For this review, use the dimensioned drawing (mm, ordinates from the lowest corner) and the shaded views. A direction names the side the tool comes from. Round coordinates to 2 decimals unless told otherwise and drop trailing zeros. Order: outer loops, then holes, each group sorted by start corner. A loop starts at its lowest first (then second) coordinate and runs counter-clockwise, first axis right, second up. Notation, with made-up numbers: (-31, -31.5) -> (5, -31.5) arc R31 cw to (5, -4.5) -> close; hole circle Ø11 at (-2.5, 31.5). An arc over 180 degrees is marked (long way). Use a Markdown table: item, result. Add a question column.
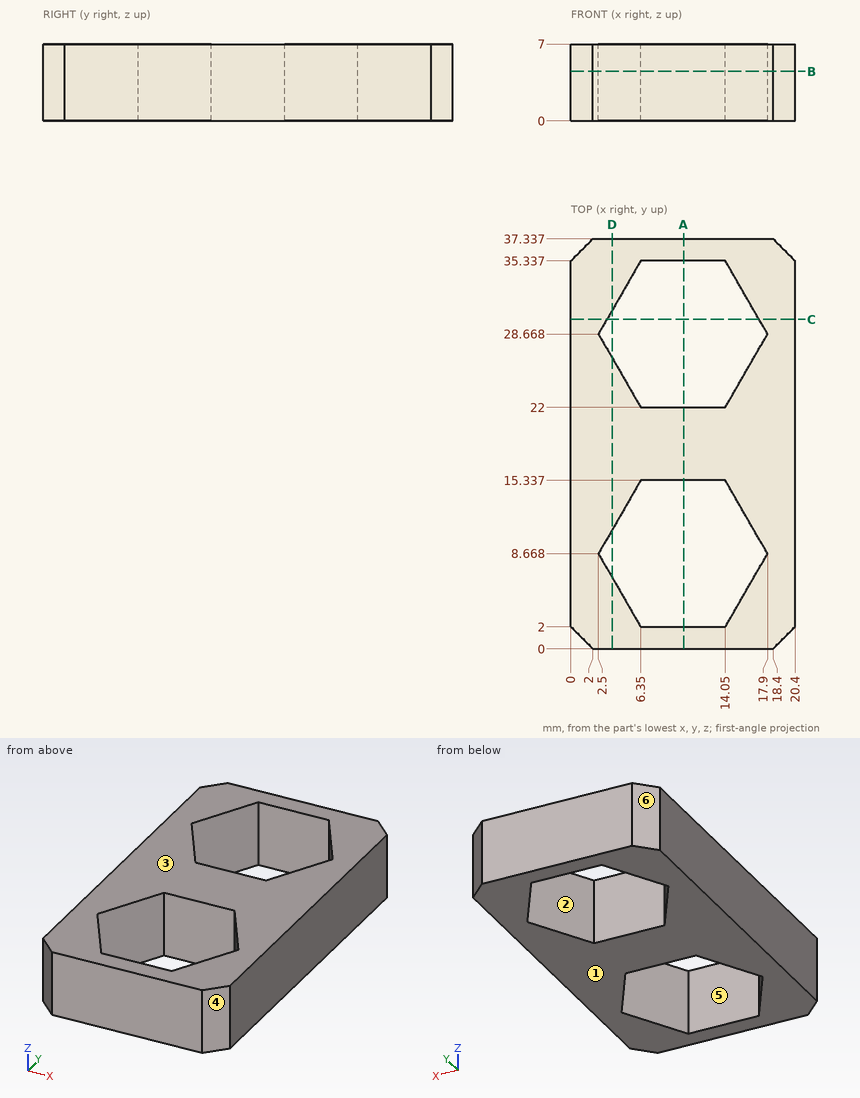
Q1. Wall thickness on line 1 (Y direction, x = 10.75, z = 4.25); line 2 (Y direction, x = 16.25, z = 6.5) (1 decimal); line 3 (X direction, y = 35, z = 2.25) (1 decimal): over which ranges is each line inside the solid? List them lowest first. Write a range as [from, to].
Q2. Add section D-D (x = 3.75). Write out the cut boundary in (y, z), then the cut area to 3 significant figures.
Q3. Add section B-B (z = 4.5). Write out the cut boundary in (x, y).
Q4. Mouldability with a two-part tool opening along X and no side actions: class the marked faces 3, 4, 5 and 6 as pulls with the +X half, pulls with the -X half, needs draft (parallel to the pull), parting line crosses it, or undercut.
Q5. Add section C-C (y = 30). Write out the cut boundary in (x, z).
Q6. Add section A-A (x = 10.25). Write out the cut boundary in (y, z).
Q7. Machinability: for the marked faces 1 and 2, which of the approach directions +Z, -Z, +X, -X, +Y, -Y give a long, thin tool a straight path to every point of the face, cutting with its end or side? Answer none if there is none.
Report:
| question | item | result |
|---|---|---|
| 1 | line 1 | y = [0, 2], [15.34, 22], [35.34, 37.34] |
| 1 | line 2 | y = [0, 5.8], [11.5, 25.8], [31.5, 37.3] |
| 1 | line 3 | x = [0, 6.2], [14.2, 20.4] |
| 2 | outline | (0, 0) -> (6.5, 0) -> (6.5, 7) -> (0, 7) -> close; (10.83, 0) -> (26.5, 0) -> (26.5, 7) -> (10.83, 7) -> close; (30.83, 0) -> (37.34, 0) -> (37.34, 7) -> (30.83, 7) -> close |
| 2 | area | 201 mm² |
| 3 | outline | (0, 2) -> (2, 0) -> (18.4, 0) -> (20.4, 2) -> (20.4, 35.34) -> (18.4, 37.34) -> (2, 37.34) -> (0, 35.34) -> close; hole (2.5, 8.67) -> (6.35, 2) -> (14.05, 2) -> (17.9, 8.67) -> (14.05, 15.34) -> (6.35, 15.34) -> close; hole (2.5, 28.67) -> (6.35, 22) -> (14.05, 22) -> (17.9, 28.67) -> (14.05, 35.34) -> (6.35, 35.34) -> close |
| 4 | face 3 | needs draft |
| 4 | face 4 | pulls with the +X half |
| 4 | face 5 | undercut |
| 4 | face 6 | pulls with the -X half |
| 5 | outline | (0, 0) -> (3.27, 0) -> (3.27, 7) -> (0, 7) -> close; (17.13, 0) -> (20.4, 0) -> (20.4, 7) -> (17.13, 7) -> close |
| 6 | outline | (0, 0) -> (2, 0) -> (2, 7) -> (0, 7) -> close; (15.34, 0) -> (22, 0) -> (22, 7) -> (15.34, 7) -> close; (35.34, 0) -> (37.34, 0) -> (37.34, 7) -> (35.34, 7) -> close |
| 7 | face 1 | -Z, +X, -X, +Y, -Y |
| 7 | face 2 | +Z, -Z |
